Could you check a few things on this drawing? It's one solid part, dimensions in mm from its lowest x, y, z. A direction names the side the tool comes from. Coordinates: 2 decimals unless noted, no trailing zeros. Loops run counter-clockwise (first coordinate to the right, second up) from the corner with the lowest first, then second, coordinate; pieces in that order, holes last. Notation, with made-up numbers: (14.5, 54.25) -> (30.5, 54.25) arc R24 ccw to (30.5, 73.25) -> close; hole circle Ø9 at (-37.75, 14). An arc over 180 degrees is marked (long way). One line per question, with ' | ' between items. Start each with the question number.
(1) If we mould it in two halves opening along X, with no side actions, what happens to the marked faces 1, 2, 3 and 4? For each: pulls with the +X half, pulls with the -X half, needs draft (parallel to the pull), parting line crosses it, or undercut.
(2) I'm going to push flat-ended pins straight in: pin 1 Ø13.5 at (x, y) = (61, 30.5) entering from +Z; pin 2 Ø8 at (x, z) = (65, 27.5) entering from -Y; pin 3 Ø21 at (x, z) = (62.5, 30) entering from +Y; pin 4 Ø1 at (x, y) = (60.5, 1) entering from +Z. Where does each tip first touch, or does it pass through?
(3) Suppose I cut it at A-A (z = 74). Please give me the cut outline in (x, y).
(4) Suppose I cut it at C-C (z = 41.5). Please give me the cut outline in (x, y), plus the area to 3 significant figures.
(5) Which directions (+Z, -Z, +X, -X, +Y, -Y) give clear straight access to the entire face, cutting with the end or side of a thin tool? Please do the marked faces 5 and 6.
(6) If I drill on line 1 along Y through (x, z) = (3.9, 75); line 2 along X through (y, z) = (6.5, 71); line 3 along Z through (x, y) = (19, 11), over which ranges is the centre line in solid material (lowest first)?
(7) Suppose I cut it at B-B (y = 25). Please give me the cut outline in (x, z), plus the area to 3 significant figures.
(8) Suppose I cut it at D-D (x = 78). Please give me the cut outline in (y, z).
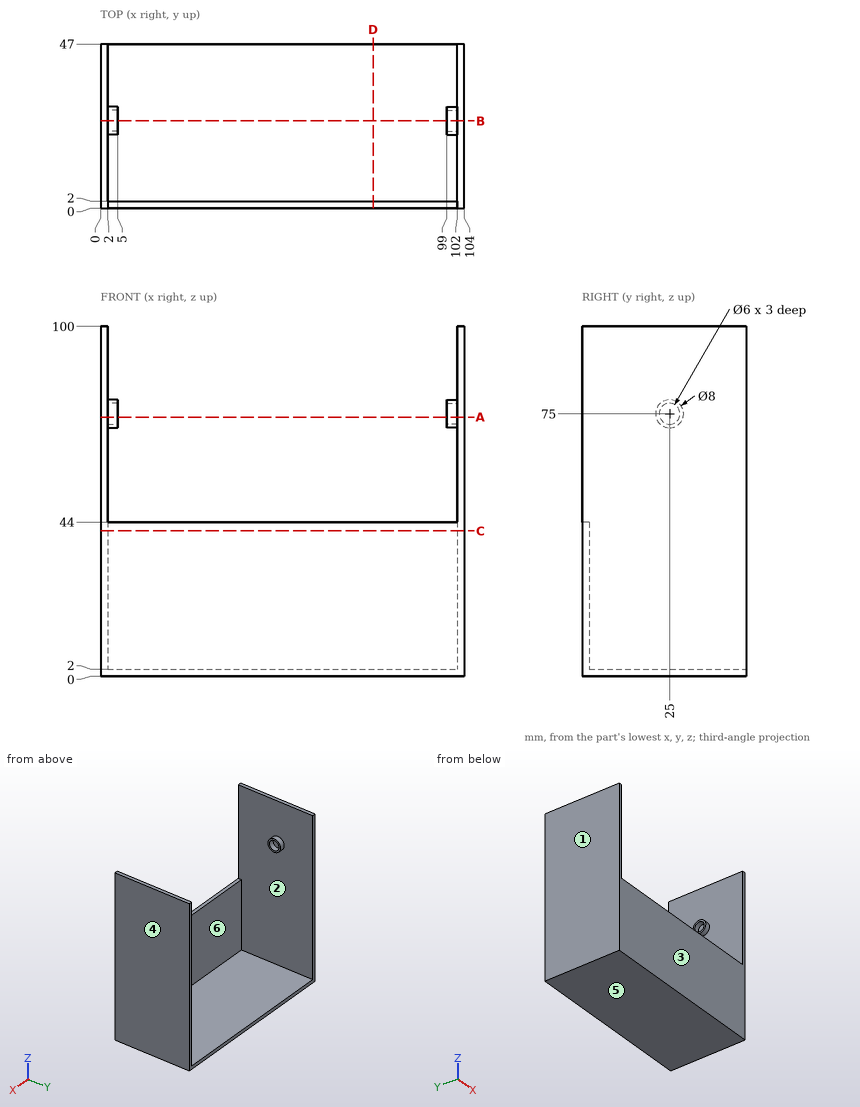
Checks:
1) face 1: pulls with the -X half | face 2: undercut | face 3: needs draft | face 4: pulls with the +X half
2) pin 1: stops at z = 2 | pin 2: stops at y = 0 | pin 3: stops at y = 2 | pin 4: stops at z = 44
3) outline: (0, 0) -> (2, 0) -> (2, 21.13) -> (5, 21.13) -> (5, 22.17) -> (2, 22.17) -> (2, 27.83) -> (5, 27.83) -> (5, 28.87) -> (2, 28.87) -> (2, 47) -> (0, 47) -> close; (99, 21.13) -> (102, 21.13) -> (102, 0) -> (104, 0) -> (104, 47) -> (102, 47) -> (102, 28.87) -> (99, 28.87) -> (99, 27.83) -> (102, 27.83) -> (102, 22.17) -> (99, 22.17) -> close
4) outline: (0, 0) -> (104, 0) -> (104, 47) -> (102, 47) -> (102, 2) -> (2, 2) -> (2, 47) -> (0, 47) -> close | area: 388 mm^2
5) face 5: -Z, +X, -X, +Y, -Y | face 6: +Z, +Y
6) line 1: y = 21 to 22, 28 to 29 | line 2: x = 0 to 2, 102 to 104 | line 3: z = 0 to 2
7) outline: (0, 0) -> (104, 0) -> (104, 100) -> (102, 100) -> (102, 79) -> (99, 79) -> (99, 78) -> (102, 78) -> (102, 72) -> (99, 72) -> (99, 71) -> (102, 71) -> (102, 2) -> (2, 2) -> (2, 71) -> (5, 71) -> (5, 72) -> (2, 72) -> (2, 78) -> (5, 78) -> (5, 79) -> (2, 79) -> (2, 100) -> (0, 100) -> close | area: 612 mm^2
8) outline: (0, 0) -> (47, 0) -> (47, 2) -> (2, 2) -> (2, 44) -> (0, 44) -> close
